from build123d import *

# Parameters (mm, degrees)
SKETCH1_R                = 36.5
BOSS_EXTRUDE1_DEPTH      = 13
SKETCH2_R                = 27.5
BOSS_EXTRUDE2_DEPTH      = 14
SKETCH3_R                = 13
BOSS_EXTRUDE3_DEPTH      = 22
SKETCH4_R                = 8
CUT_EXTRUDE1_DEPTH       = 72.172326083
BOSS_EXTRUDE4_DEPTH      = 22
BOSS_EXTRUDE4_DEPTH_BACK = 94
SKETCH6_R                = 6
SKETCH8_RX               = 22.241182767
SKETCH8_RY               = 20.063201952
CUT_EXTRUDE2_DEPTH       = 13
SKETCH10_R               = 4.5
CUT_EXTRUDE3_DEPTH       = 132.107780243


with BuildPart() as part:
    # Sketch1 → Boss-Extrude1 (new body)
    with BuildSketch(Plane.XY):
        with Locations(Location((0, 0, 0), (0, 0, 180))):
            Circle(SKETCH1_R)
    extrude(amount=BOSS_EXTRUDE1_DEPTH)

    # Sketch2 → Boss-Extrude2 (add)
    with BuildSketch(Plane.XY.offset(13)):
        Circle(SKETCH2_R)
    extrude(amount=BOSS_EXTRUDE2_DEPTH)

    # Sketch3 → Boss-Extrude3 (add)
    with BuildSketch(Plane.XY.offset(27)):
        Circle(SKETCH3_R)
    extrude(amount=BOSS_EXTRUDE3_DEPTH)

    # Sketch4 → Cut-Extrude1 (cut, through all)
    with BuildSketch(Plane.XY.offset(49)):
        Circle(SKETCH4_R)
    extrude(amount=-CUT_EXTRUDE1_DEPTH, mode=Mode.SUBTRACT)

    # Sketch6 → Boss-Extrude4 (add, two sides: drawn at the far end of the back side and taken through both)
    with BuildSketch(Plane(origin=(36.5, 0, 0), x_dir=(0, 0, -1), z_dir=(1, 0, 0)).offset(-BOSS_EXTRUDE4_DEPTH_BACK)):
        with Locations((-16.5, 12.5)):
            Circle(SKETCH6_R)
    extrude(amount=BOSS_EXTRUDE4_DEPTH + BOSS_EXTRUDE4_DEPTH_BACK)

    # Sketch8 → Cut-Extrude2 (cut)
    with BuildSketch(Plane(origin=(0, 0, 0), x_dir=(-1, 0, 0), z_dir=(0, 0, -1))):
        with Locations((0, 0)):
            Ellipse(SKETCH8_RX, SKETCH8_RY)
    extrude(amount=-CUT_EXTRUDE2_DEPTH, mode=Mode.SUBTRACT)

    # Sketch10 → Cut-Extrude3 (cut, through all)
    with BuildSketch(Plane(origin=(58.5, 0, 0), x_dir=(0, 0, -1), z_dir=(1, 0, 0))):
        with Locations((-16.5, 12.5)):
            Circle(SKETCH10_R)
    extrude(amount=-CUT_EXTRUDE3_DEPTH, mode=Mode.SUBTRACT)


solid = part.part
Geometry: final body of the model. Coordinates: model frame, mm. A direction names the side the tool comes from. Round coordinates to 2 decimals unless told otherwise and drop trailing zeros. Order: outer loops, then holes, each group sorted by start corner. A loop starts at its lowest first (then second) coordinate and runs counter-clockwise, first axis right, second up. Notation, with made-up numbers: (67, -36.5) -> (99, -36.5) arc R23 cw to (99, -27.5) -> close; hole circle Ø11 at (-31, 73). An arc over 180 degrees is marked (long way). Put each result on its own line as item: value. Start each with the question number.
Q1. Section C-C on z = 41.5. Return the cut outline in (x, y), and give its area (3 significant figures).
Q2. First-contact query: pin 1 (16.5 mm diameter, centred on x = -12.5, y = -5.5, fed in from +Z); pin 2 (10 mm diameter, centred on x = -9.5, y = 8, fed in from -Z); pin 3 (1 mm diameter, centred on x = -24.5, y = 24, fed in from +Z); pin 4 (15.5 mm diameter, centred on x = -15.5, y = 30, fed in from +Z). Flat tips, straight axial feed; report the tip coordinate or a pass-through.
Q3. Reachability of faces 1 (the cylindrical face through (-0.07, 6.51, 16.86)), 2 (the cylindrical face through (-10.316, -7.91, 37.846)), 3 (the flat face through (-57.5, 17, 14)) from +Z, -Z, +X, -X, +Y, -Y: full face, straight path, thin tool, end or side. Return the list, or none.
Q4. Pull-direction query (Z, two-part tool) for faces 4 (the flat face through (-16, 16, 0)), 5 (the flat face through (6, -12, 27)), 6 (the flat face through (58.5, 17, 14)), 7 (the cylindrical face through (1.312, 12.698, 20.996)); classes: +Z half, -Z half, draft (parallel to the pull), parting line (faces both ways), or undercut.
Q5. Section B-B on x = 44.5. Return the cut outline in (y, z), and give its area (3 significant figures).
Q6. Section A-A on z = 16.5. Return the cut outline in (x, y), and give its area (3 significant figures).
Q7. Line query: probe 1 along X at (y, z) = (-0.5, 11); probe 2 along Y at (x, z) = (0, 27.5); probe 3 along X at (y, z) = (0, 23). Output: solid intervals per line, ascending.
Q8. Section D-D on y = 32.5. Return the cut outline in (x, z), and give its area (3 significant figures).
Ans:
1. outline: circle Ø26 at (0, 0); hole circle Ø16 at (0, 0)
1. area: 330 mm2
2. pin 1: stops at z = 49
2. pin 2: stops at z = 13
2. pin 3: stops at z = 13
2. pin 4: stops at z = 27
3. face 1: none
3. face 2: +Z
3. face 3: +Z, -Z, -X, +Y, -Y
4. face 4: -Z half
4. face 5: +Z half
4. face 6: draft
4. face 7: undercut
5. outline: circle Ø12 at (12.5, 16.5); hole circle Ø9 at (12.5, 16.5)
5. area: 49.5 mm2
6. outline: (-57.5, 6.5) -> (-26.72, 6.5) arc R27.5 ccw (long way) to (26.72, 6.5) -> (58.5, 6.5) -> (58.5, 8) -> (-57.5, 8) -> close; (-57.5, 17) -> (58.5, 17) -> (58.5, 18.5) -> (20.35, 18.5) arc R27.5 ccw to (-20.35, 18.5) -> (-57.5, 18.5) -> close; hole (-4.66, 6.5) arc R8 ccw (long way) to (4.66, 6.5) -> close
6. area: 1,950 mm2
7. probe 1: x = -36.5 to -22.23, 22.23 to 36.5
7. probe 2: y = -13 to -8, 8 to 13
7. probe 3: x = -27.5 to -8, 8 to 27.5
8. outline: (-16.61, 0) -> (16.61, 0) -> (16.61, 13) -> (-16.61, 13) -> close
8. area: 432 mm2
